Drawing for the job (mm, zero at the part's lowest x, y, z). A direction names the side the tool comes from. Give positions to 0.01 mm unless a question says otherwise; leave off trailing zeros. Write each loop counter-clockwise with the first axis right and the second up, starting at its lowest first coordinate (ties: lowest second). Pieces come first, ordered by that corner, then holes. Notation, with made-up numbers: M 11.25,-16.75 L 17.25,-16.75 A20 cw 17.25,21.25 Z; hole C 80.5,49.25 d8. An arc over 180 degrees is marked long. Answer as a JSON object with one key per item and string values. Group by question number.
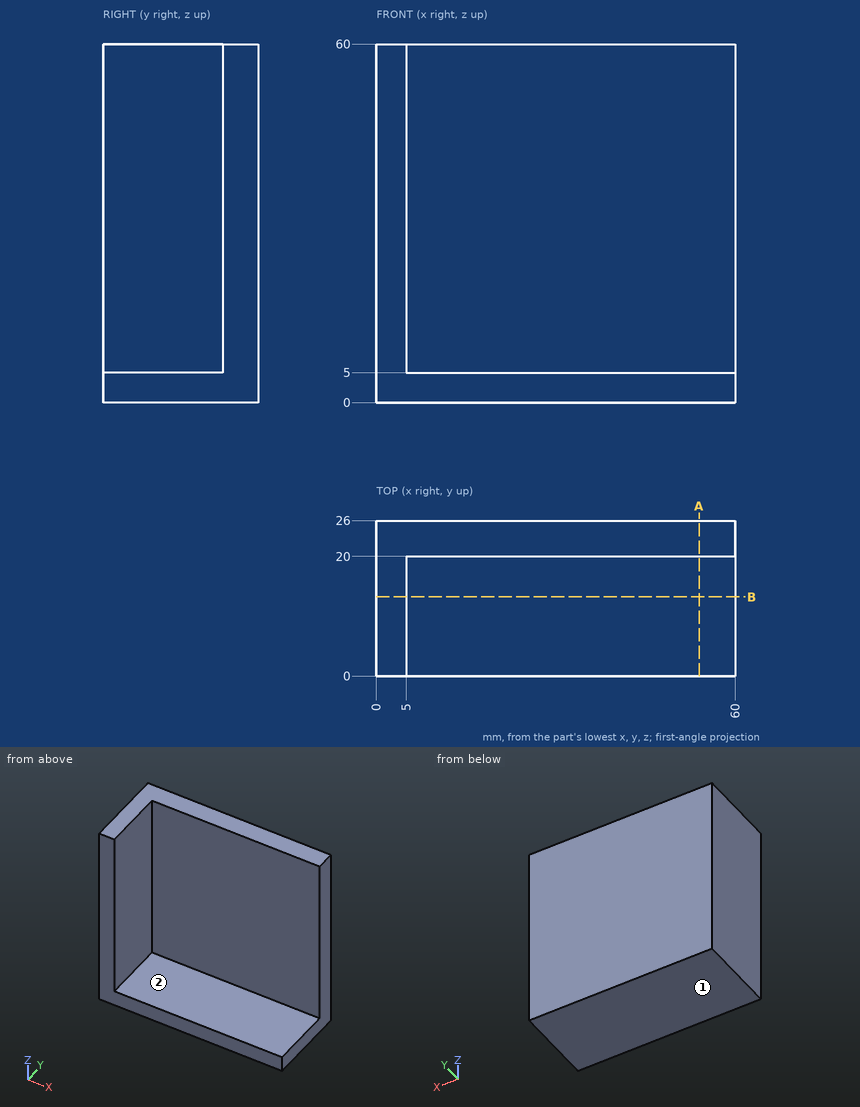
Q1. Slice it at B-B, the plane y = 13.25. Write the cut outline in (x, z).
Q2. Drop flat-ended pins along their axis: P1, Ø10, axis at x = 23.5, y = 11, coming from the +Z side; P2, Ø5, axis at x = 31, z = 51, coming from the -Y side; P3, Ø10, axis at y = 10, z = 19, coming from the +X side. Give the stop position or say it passes through.
Q3. Wall check: L1, parallel to X at y = 10, z = 42.5; L2, parallel to Y at x = 8, z = 18.5. Give the ranges that are in metal, low to high.
Q4. 3-axis set-ups, long thin cutter, end or side, ignore diameter. For the marked faces 1 and 2: which of +Z, -Z, +X, -X, +Y, -Y reach the whole face in a straight line?
Q5. Slice it at A-A, the plane x = 54. Write the cut outline in (y, z), then the cut area to 3 significant figures.
Solved:
{
 "1": {"outline": "M 0,0 L 60,0 L 60,5 L 5,5 L 5,60 L 0,60 Z"},
 "2": {"P1": "stops at z = 5", "P2": "stops at y = 20", "P3": "stops at x = 5"},
 "3": {"L1": "x = 0 to 5", "L2": "y = 20 to 26"},
 "4": {"face 1": "-Z, +X, -X, +Y, -Y", "face 2": "+Z, +X, -Y"},
 "5": {"outline": "M 0,0 L 26,0 L 26,60 L 20,60 L 20,5 L 0,5 Z", "area": "460 mm²"}
}
